Input: part model. Units: mm. Frame: model coordinates. Round coordinates to 2 decimals unless told otherwise and drop trailing zeros. Order: outer loops, then holes, each group sorted by start corner. A loop starts at its lowest first (then second) coordinate and runs counter-clockwise, first axis right, second up. Notation, with made-up numbers: M 84.25,86 L 133.25,86 A11 ccw 133.25,95 Z; hole C 4,-1.5 d1. An arc over 180 degrees is marked long. One line per question, with ' | ' between items.
```python
from build123d import *

# Parameters (mm, degrees)
BOSS_EXTRUDE1_DEPTH = 3
SKETCH2_R           = 4.3
CUT_EXTRUDE1_DEPTH  = 148.721020847


with BuildPart() as part:
    # Sketch1 → Boss-Extrude1 (new body)
    with BuildSketch(Plane.XY):
        with BuildLine():
            Line((0, 7.5), (140, 7.5))
            ThreePointArc((140, 7.5), (147.5, 0), (140, -7.5))
            Line((140, -7.5), (0, -7.5))
            ThreePointArc((0, -7.5), (-7.5, 0), (0, 7.5))
        make_face()
    extrude(amount=BOSS_EXTRUDE1_DEPTH)

    # Sketch2 → Cut-Extrude1 (cut, through all)
    with BuildSketch(Plane.XY.offset(3)):
        Circle(SKETCH2_R)
        with Locations((140, 0)):
            Circle(SKETCH2_R)
        with Locations((63.1, 0)):
            Circle(SKETCH2_R)
    extrude(amount=-CUT_EXTRUDE1_DEPTH, mode=Mode.SUBTRACT)


solid = part.part
```
Item 1: Section query A-A, the plane z = 2.1. Return loops of the section in (x, y), plus the area to 3 significant figures.
Report:
outline: M 0,-7.5 L 140,-7.5 A7.5 ccw 140,7.5 L 0,7.5 A7.5 ccw Z; hole C 0,0 d8.6; hole C 63.1,0 d8.6; hole C 140,0 d8.6 | area: 2,100 mm²
Item 2: Line query: line 1 along Y through (x, z) = (63.1, 1.6); line 2 along X through (y, z) = (-1, 0.2); line 3 along X through (y, z) = (-1.5, 1.65). Output: solid intervals per line, ascending. Write a range as from..to.
Report:
line 1: -7.5..-4.3, 4.3..7.5 | line 2: -7.43..-4.18, 4.18..58.92, 67.28..135.82, 144.18..147.43 | line 3: -7.35..-4.03, 4.03..59.07, 67.13..135.97, 144.03..147.35
Item 3: Section query B-B, the plane x = 66. Return loops of the section in (y, z).
Report:
outline: M -7.5,0 L -3.17,0 L -3.17,3 L -7.5,3 Z; M 3.17,0 L 7.5,0 L 7.5,3 L 3.17,3 Z
Item 4: Mould query, pull axis Y, two halves, no side actions, for faces 1 (the cylindrical face through (147.5, 0.16, 1.48)), 2 (the cylindrical face through (-4.296, 0.189, 1.521)), 3 (the flat face through (71, 0, 3)). Classes: +Y half, -Y half, draft (parallel to the pull), parting line (faces both ways), or undercut.
Report:
face 1: parting line | face 2: undercut | face 3: draft
Item 5: First-contact query: pin 1 (1.5 mm diameter, centred on y = 3, z = 2, fed in from +X). Flat tip, straight axial feed; report the tip coordinate or a pass-through.
Report:
pin 1: x = 147.15
